Could you check a few things on this model? Use its own coordinates, in mm. A direction names the side the tool comes from. Round coordinates to 2 decimals unless told otherwise and drop trailing zeros. Loops run counter-clockwise (first coordinate to the right, second up) from the corner with the lowest first, then second, coordinate; pieces in that order, holes last. Notation, with made-up numbers: (-36, 39.5) -> (9, 39.5) arc R20 cw to (9, 56.5) -> close; hole circle Ø10 at (87, -5). An arc over 180 degrees is marked (long way). Write each question's results on one line, items separated by ' | '.
from build123d import *

# Parameters (mm, degrees)
F1_DEPTH = 76.2
F2_R     = 12.7
F3_DEPTH = 76.201
F5_DEPTH = 17.9342755506
F7_DEPTH = 25.401


# Not quite as in the source:
# - a pattern or mirror of a feature is missing from the dataset's text; its kind, count and spacing are read off the source's solid


with BuildPart() as f1:
    # F0 (on Front) → F1 (new body, symmetric)
    with BuildSketch(Plane.XZ):
        Polygon((0, 0), (0, 152.4), (-25.4, 152.4), (-25.4, 17.9332755506), (-76.2, 17.9332755506), (-76.2, 0), align=None)
    extrude(amount=F1_DEPTH, both=True)

    # F2 (on face) → F3 (cut, through all)
    with BuildSketch(Plane.YZ):
        with Locations((0, 101.6)):
            Circle(F2_R)
    extrude(amount=-F3_DEPTH, mode=Mode.SUBTRACT)

    # F4 (on face) → F5 (cut, through all)
    with BuildSketch(Plane.XY.offset(17.9332755506)):
        with BuildLine():
            Line((-63.5, 12.7), (-76.2, 12.7))
            Line((-76.2, 12.7), (-76.2, -12.7))
            Line((-76.2, -12.7), (-63.5, -12.7))
            ThreePointArc((-63.5, -12.7), (-50.8, 0), (-63.5, 12.7))
        make_face()
    extrude(amount=-F5_DEPTH, mode=Mode.SUBTRACT)

    # F6 (on face) → F7 (cut, through all)
    with BuildSketch(Plane(origin=(-25.4, 0, 0), x_dir=(0, -1, 0), z_dir=(-1, 0, 0))):
        with BuildLine():
            ThreePointArc((-76.2, 114.3), (-65.0407683632, 141.2407683632), (-38.1, 152.4))
            Line((-38.1, 152.4), (-76.2, 152.4))
            Line((-76.2, 152.4), (-76.2, 114.3))
        make_face()
    f7 = extrude(amount=-F7_DEPTH, mode=Mode.SUBTRACT)

    # F7_copies: F7 across plane
    add(f7.mirror(Plane(origin=(0, 0, 0), x_dir=(0, 0, -1), z_dir=(0, -1, 0))), mode=Mode.SUBTRACT)


solid = f1.part
1) I want a section at A-A, the plane y = 0. Write out the boundary of the cut face in (x, z), plus the area to 3 significant figures.
Model answer:
outline: (-50.8, 0) -> (0, 0) -> (0, 88.9) -> (-25.4, 88.9) -> (-25.4, 17.93) -> (-50.8, 17.93) -> close; (-25.4, 114.3) -> (0, 114.3) -> (0, 152.4) -> (-25.4, 152.4) -> close | area: 3,680 mm2
2) If we mould it in two halves opening along Y, with no side actions, what happens to faces 1 (the flat face through (-70, 12.7, 9)), 2 (the flat face through (-25.4, -1, 86)), 3 (the cylindrical face through (-12.88, -65.34, 140.94)), 4 (the cylindrical face through (-12.88, 65.34, 140.94))? For each: released by +Y, released by -Y, zero draft, split by the parting line, or undercut.
Model answer:
face 1: undercut | face 2: zero draft | face 3: released by -Y | face 4: released by +Y
3) I want a section at D-D, the plane y = -32. Write out the boundary of the cut face in (x, z).
Model answer:
outline: (-76.2, 0) -> (0, 0) -> (0, 152.4) -> (-25.4, 152.4) -> (-25.4, 17.93) -> (-76.2, 17.93) -> close
4) I need wall thicknesses on line 1 (Z direction, x = -18, y = 0); line 2 (Y direction, x = -20, z = 101); line 3 (X direction, y = -59, z = 112.5). Which ranges of each line are inside material? Lowest first, please.
Model answer:
line 1: z = 0 to 88.9, 114.3 to 152.4 | line 2: y = -76.2 to -12.69, 12.69 to 76.2 | line 3: x = -25.4 to 0
5) I want a section at B-B, the plane z = 101.6. Write out the boundary of the cut face in (x, y).
Model answer:
outline: (-25.4, -76.2) -> (0, -76.2) -> (0, -12.7) -> (-25.4, -12.7) -> close; (-25.4, 12.7) -> (0, 12.7) -> (0, 76.2) -> (-25.4, 76.2) -> close
6) I'm going to push flat-ended pins straight in: pin 1 (1 mm diameter, centred on y = -3.5, z = 20.5, fed in from +X); pin 2 (4 mm diameter, centred on y = -26.5, z = 121, fed in from -X); pin 3 (5 mm diameter, centred on x = -42.5, y = -9.5, fed in from +Z); pin 4 (15 mm diameter, centred on y = 0, z = 101.6, fed in from -X). Where does each tip first touch, or does it pass through?
Model answer:
pin 1: stops at x = 0 | pin 2: stops at x = -25.4 | pin 3: stops at z = 17.93 | pin 4: passes through
7) I want a section at C-C, the plane x = -11. Write out the boundary of the cut face in (y, z), plus the area to 3 significant figures.
Model answer:
outline: (-76.2, 0) -> (76.2, 0) -> (76.2, 114.3) arc R38.1 ccw to (38.1, 152.4) -> (-38.1, 152.4) arc R38.1 ccw to (-76.2, 114.3) -> close; hole circle Ø25.4 at (0, 101.6) | area: 22,100 mm2
8) For faces 5 (the flat face through (-50, -1, 17.933)), 6 (the flat face through (-70, -12.7, 9)), 7 (the flat face through (-22, -76.2, 45)), which set-ups out of +Z, -Z, +X, -X, +Y, -Y let a thin tool reach every point of the face, with its end or its side?
Model answer:
face 5: +Z, -X, +Y, -Y | face 6: +Z, -Z, -X | face 7: +Z, -Z, +X, -X, -Y
